For this review, take the finished solid that the model builds, in its own axes (mm). Face numbers are marked on the shaded views. A direction names the side the tool comes from. Round coordinates to 2 decimals unless told otherwise and drop trailing zeros. Order: outer loops, then holes, each group sorted by start corner. A loop starts at its lowest first (then second) coordinate and runs counter-clockwise, first axis right, second up. Notation, with made-up numbers: (53, 69) -> (106, 69) arc R18 ccw to (106, 86) -> close; hole circle Ø2 at (64, 59.5). An arc over 180 degrees is marked (long way). Use a Markdown table: item, result. Add a question column.
1) Consider section A-A (y = 27). State the section outline as (x, z) points, plus the area to 3 significant figures.
2) Clearance check with flat-ended pins moving along their axes: P1, Ø3.5, axis at x = 9, y = 76, coming from the -Z side; P2, Ø2, axis at y = 42.5, z = 7, coming from the +X side; P3, Ø6, axis at x = 9, y = 43.5, coming from the +Z side. State where each tip first meets the part, or that it passes through.
3) Consider section C-C (y = 76). State the section outline as (x, z) points.
4) Consider section B-B (x = 9). State the section outline as (y, z) points.
5) Wall thickness on line 1 along Y through (x, z) = (9, 1.35); line 2 along Y through (x, z) = (8, 1.25); line 3 along Z through (x, y) = (2.25, 46): over which ranges is each line inside the solid? List them lowest first. Write a range as [from, to].
6) Machinability: for the marked faces 1 and 2, which of the approach directions +Z, -Z, +X, -X, +Y, -Y give a long, thin tool a straight path to every point of the face, cutting with its end or side? Answer none if there is none.
```python
from build123d import *

# Parameters (mm, degrees)
SKETCH001_W  = 50
SKETCH001_H  = 3
PAD001_DEPTH = 3
SKETCH_R     = 2.1
PAD_DEPTH    = 3


with BuildPart() as pad001:
    # Sketch001 → Pad001 (new body)
    with BuildSketch(Plane.YZ):
        Polygon((0, 0), (82, 0), (82, 8), (78, 10.001209), (4, 10.001209), (0, 8), align=None)
        with Locations((42.5338, 4.983344)):
            Rectangle(SKETCH001_W, SKETCH001_H, mode=Mode.SUBTRACT)
    extrude(amount=PAD001_DEPTH)


with BuildPart() as fusion:
    # Sketch → Pad (new body)
    with BuildSketch(Plane.XY):
        Polygon((0, 82), (0, 0), (9.787406, 0), (14.999606, 4), (14.999606, 78), (9.787406, 82), align=None)
        with Locations((9, 6)):
            Circle(SKETCH_R, mode=Mode.SUBTRACT)
        with Locations((9, 76)):
            Circle(SKETCH_R, mode=Mode.SUBTRACT)
    extrude(amount=PAD_DEPTH)

    # Fusion: union Pad001
    add(pad001.part)


solid = fusion.part
```
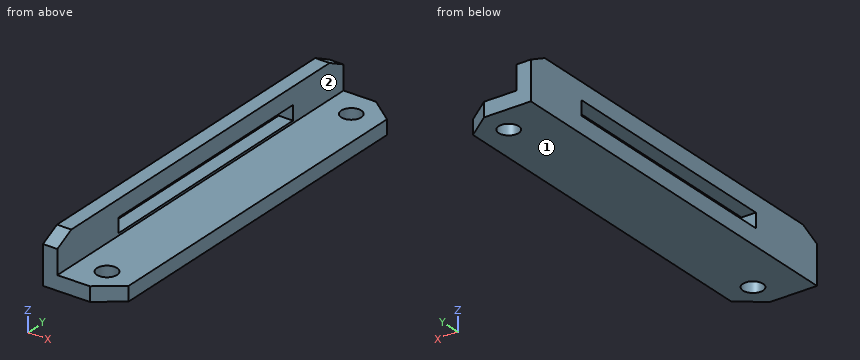
Results list:
| question | item | result |
|---|---|---|
| 1 | outline | (0, 0) -> (15, 0) -> (15, 3) -> (3, 3) -> (3, 3.48) -> (0, 3.48) -> close; (0, 6.48) -> (3, 6.48) -> (3, 10) -> (0, 10) -> close |
| 1 | area | 57.0 mm2 |
| 2 | P1 | through |
| 2 | P2 | x = 3 |
| 2 | P3 | z = 3 |
| 3 | outline | (0, 0) -> (6.9, 0) -> (6.9, 3) -> (3, 3) -> (3, 10) -> (0, 10) -> close; (11.1, 0) -> (15, 0) -> (15, 3) -> (11.1, 3) -> close |
| 4 | outline | (0, 0) -> (3.9, 0) -> (3.9, 3) -> (0, 3) -> close; (8.1, 0) -> (73.9, 0) -> (73.9, 3) -> (8.1, 3) -> close; (78.1, 0) -> (82, 0) -> (82, 3) -> (78.1, 3) -> close |
| 5 | line 1 | [0, 3.9], [8.1, 73.9], [78.1, 82] |
| 5 | line 2 | [0, 4.15], [7.85, 74.15], [77.85, 82] |
| 5 | line 3 | [0, 3.48], [6.48, 10] |
| 6 | face 1 | -Z, +X, -X, +Y, -Y |
| 6 | face 2 | +Z, +X, +Y, -Y |
